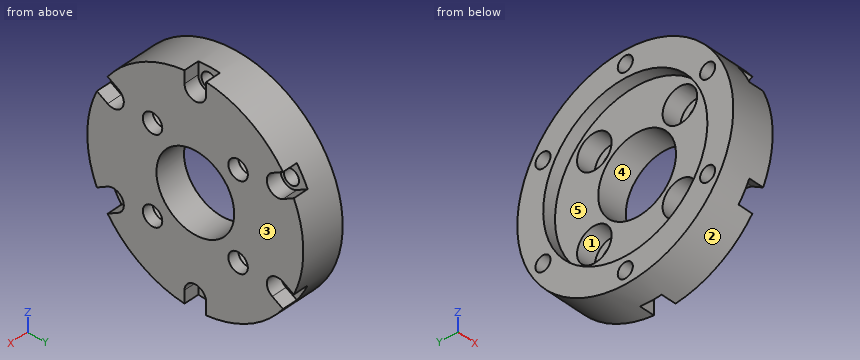
```python
from build123d import *

# Parameters (mm, degrees)
ENL_V_MAT_EXTRU_1_DEPTH                         = 3.5
R_P_TITION_CIRCULAIRE1_COUNT                    = 6
ESQUISSE3_R                                     = 1.75
ENL_V_MAT_EXTRU_2_DEPTH                         = 36.947878936
R_P_TITION_CIRCULAIRE2_COUNT                    = 6
CHAMBRAGE_POUR_VIS_T_TE_CYLINDRIQUE_D           = 4.5
CHAMBRAGE_POUR_VIS_T_TE_CYLINDRIQUE_CBORE_D     = 8
CHAMBRAGE_POUR_VIS_T_TE_CYLINDRIQUE_CBORE_DEPTH = 4.5
R_P_TITION_CIRCULAIRE3_COUNT                    = 4


with BuildPart() as part:
    # Esquisse1 → Base-Révolution (revolve)
    with BuildSketch(Plane.XY, mode=Mode.PRIVATE) as base_r_volution_sk:
        Polygon((-5, 25), (-5, 19), (-2, 19), (-2, 9), (5, 9), (5, 25), align=None)
    revolve(base_r_volution_sk.sketch.rotate(Axis((-14.936373376, 0, 0), (1, 0, 0)), 90), axis=Axis((-14.936373376, 0, 0), (1, 0, 0)))

    # Esquisse2 → Enlèv. mat.-Extru.1 (cut)
    with BuildSketch(Plane(origin=(5, 0, 0), x_dir=(0, 0, -1), z_dir=(1, 0, 0))):
        with BuildLine():
            Line((-22, 2.5), (-25.435164017, 2.5))
            Line((-25.435164017, 2.5), (-25.435164017, -2.5))
            Line((-25.435164017, -2.5), (-22, -2.5))
            ThreePointArc((-22, -2.5), (-19.5, 0), (-22, 2.5))
        make_face()
    enl_v_mat_extru_1 = extrude(amount=-ENL_V_MAT_EXTRU_1_DEPTH, mode=Mode.SUBTRACT)

    # Répétition circulaire1: Enlèv. mat.-Extru.1 ×6 about axis
    r_p_tition_circulaire1_axis = Axis((0, 0, 0), (1, 0, 0))
    for i in range(1, R_P_TITION_CIRCULAIRE1_COUNT):
        add(enl_v_mat_extru_1.rotate(r_p_tition_circulaire1_axis, i * 360 / R_P_TITION_CIRCULAIRE1_COUNT), mode=Mode.SUBTRACT)

    # Esquisse3 → Enlèv. mat.-Extru.2 (cut, through all)
    with BuildSketch(Plane(origin=(1.5, 0, 0), x_dir=(0, 0, -1), z_dir=(1, 0, 0))):
        with Locations((-22, 0)):
            Circle(ESQUISSE3_R)
    enl_v_mat_extru_2 = extrude(amount=-ENL_V_MAT_EXTRU_2_DEPTH, mode=Mode.SUBTRACT)

    # Répétition circulaire2: Enlèv. mat.-Extru.2 ×6 about axis
    r_p_tition_circulaire2_axis = Axis((0, 0, 0), (1, 0, 0))
    for i in range(1, R_P_TITION_CIRCULAIRE2_COUNT):
        add(enl_v_mat_extru_2.rotate(r_p_tition_circulaire2_axis, i * 360 / R_P_TITION_CIRCULAIRE2_COUNT), mode=Mode.SUBTRACT)

    # Chambrage pour vis à tête cylindrique à 6 pans creux (vis CHC) M41 (through all)
    with Locations(Plane.ZY.offset(2)):
        with Locations((9.899494937, 9.899494937)):
            chambrage_pour_vis_t_te_cylindrique = CounterBoreHole(CHAMBRAGE_POUR_VIS_T_TE_CYLINDRIQUE_D / 2, CHAMBRAGE_POUR_VIS_T_TE_CYLINDRIQUE_CBORE_D / 2, CHAMBRAGE_POUR_VIS_T_TE_CYLINDRIQUE_CBORE_DEPTH)

    # Répétition circulaire3: Chambrage pour vis à tête cylindrique à 6 pans creux (vis CHC) M41 ×4 about axis
    r_p_tition_circulaire3_axis = Axis((0, 0, 0), (1, 0, 0))
    for i in range(1, R_P_TITION_CIRCULAIRE3_COUNT):
        add(chambrage_pour_vis_t_te_cylindrique.rotate(r_p_tition_circulaire3_axis, i * 360 / R_P_TITION_CIRCULAIRE3_COUNT), mode=Mode.SUBTRACT)


solid = part.part
```
Work out the finished part from the listing and answer in its coordinate system (mm). Face numbers are marked on the shaded views. A direction names the side the tool comes from. Give positions to 0.01 mm unless a question says otherwise; leave off trailing zeros. Order: outer loops, then holes, each group sorted by start corner. A loop starts at its lowest first (then second) coordinate and runs counter-clockwise, first axis right, second up. Notation, with made-up numbers: M -23,6 L -15,6 A12 cw -15,10 Z; hole C -24.5,-12.5 d10. An arc over 180 degrees is marked long. Return JSON: item names as keys, results as strings.
1) For a pull along Y with two mould halves and no side action, classify the marked faces 1, 2 and 3 as +Y half, -Y half, draft (parallel to the pull), parting line (faces both ways), or undercut.
Resolved:
{"face 1": "undercut", "face 2": "parting line", "face 3": "draft"}
2) Straight lines are drawn through the part: line 1 along Z through (x, y) = (0.25, 12); line 2 along Z through (x, y) = (-3.5, 0.5) (3 decimals); line 3 along Z through (x, y) = (-3.25, 1.5). For each, find the intervals that lie inside material, in ascending order. Write a range as [from, to].
Resolved:
{"line 1": "[-21.93, -13.3], [-6.5, 6.5], [13.3, 21.93]", "line 2": "[-24.995, -23.677], [-20.323, -18.993], [18.993, 20.323], [23.677, 24.995]", "line 3": "[-24.95, -22.9], [-21.1, -18.94], [18.94, 21.1], [22.9, 24.95]"}
3) Section D-D, the plane y = -5 is taken. Write down the section's boundary in (x, z), plus the area to 3 significant figures.
Resolved:
{"outline": "M -5,-24.49 L 5,-24.49 L 5,-7.48 L -2,-7.48 L -2,-18.33 L -5,-18.33 Z; M -5,18.33 L -2,18.33 L -2,7.48 L 5,7.48 L 5,24.49 L -5,24.49 Z", "area": "275 mm^2"}
4) A tool of negligible diameter and unlimited length cuts with its end or side. For the marked faces 4 and 5, from which of +Z, -Z, +X, -X, +Y, -Y can it reach the whole face along a straight path? Write none if from no direction.
Resolved:
{"face 4": "+X, -X", "face 5": "-X"}
5) Section B-B, the plane z = 0 is taken. Write down the section's boundary in (x, y).
Resolved:
{"outline": "M -5,-25 L 5,-25 L 5,-9 L -2,-9 L -2,-19 L -5,-19 Z; M -5,19 L -2,19 L -2,9 L 5,9 L 5,25 L -5,25 Z"}
6) Section C-C, the plane x = -3.5 is taken. Write down the section's boundary in (y, z) (3 decimals).
Resolved:
{"outline": "C 0,0 d50; hole C -19.053,-11 d3.5; hole C -19.053,11 d3.5; hole C 0,0 d38; hole C 0,-22 d3.5; hole C 0,22 d3.5; hole C 19.053,-11 d3.5; hole C 19.053,11 d3.5"}
7) Section A-A, the plane y = 0 is taken. Write down the section's boundary in (x, z), plus the area to 3 significant figures.
Resolved:
{"outline": "M -5,-25 L 1.5,-25 L 1.5,-23.75 L -5,-23.75 Z; M -5,-20.25 L 1.5,-20.25 L 1.5,-19.5 L 5,-19.5 L 5,-9 L -2,-9 L -2,-19 L -5,-19 Z; M -5,19 L -2,19 L -2,9 L 5,9 L 5,19.5 L 1.5,19.5 L 1.5,20.25 L -5,20.25 Z; M -5,23.75 L 1.5,23.75 L 1.5,25 L -5,25 Z", "area": "176 mm^2"}
8) Each of these flat-tipped pins is pushed along its axis until it touches: pin 1 (2 mm diameter, centred on y = 3, z = 17.5, fed in from -X); pin 2 (1.8 mm diameter, centred on y = 20.5, z = -11.5, fed in from +X); pin 3 (3 mm diameter, centred on x = 4, z = -24, fed in from +Y); pin 4 (3.5 mm diameter, centred on y = 9.9, z = 9.9, fed in from +X). Where does it stop, or does it pass through?
Resolved:
{"pin 1": "x = -2", "pin 2": "x = 1.5", "pin 3": "y = 10.9", "pin 4": "through"}
